The model under review builds one solid part; all positions refer to its coordinate system, in mm. Face numbers are marked on the shaded views. A direction names the side the tool comes from. Coordinates: 2 decimals unless noted, no trailing zeros. Order: outer loops, then holes, each group sorted by start corner. A loop starts at its lowest first (then second) coordinate and runs counter-clockwise, first axis right, second up.
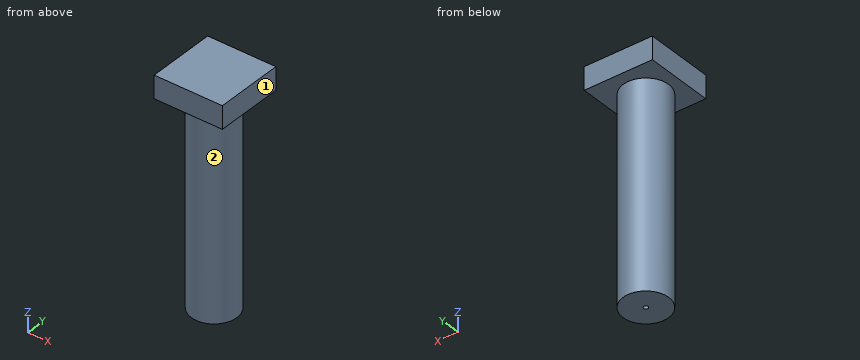
```python
from build123d import *

# Parameters (mm, degrees)
F0_W     = 7.62
F0_H     = 7.62
F1_DEPTH = 2.54
F2_R     = 1.27
F3_DEPTH = 22.86
F4_R     = 0.254
F5_DEPTH = 2.54
F2_R_2   = 2.54
F6_DEPTH = 22.86


# Not quite as in the source:
# - a feature names something its author has since deleted; it is built from what else it names


with BuildPart() as f1:
    # F0 (on Top) → F1 (new body)
    with BuildSketch(Plane.XY):
        with Locations((-38.7955456972, -21.8359371471)):
            Rectangle(F0_W, F0_H)
    extrude(amount=F1_DEPTH)

    # F2 (on face) → F3 (join)
    with BuildSketch(Plane(origin=(0, 0, 0), x_dir=(1, 0, 0), z_dir=(0, 0, -1))):
        with Locations((-38.854431361, 21.8882076442)):
            Circle(F2_R)
    extrude(amount=F3_DEPTH)

    # F4 (on face) → F5 (cut)
    with BuildSketch(Plane(origin=(0, 0, -22.86), x_dir=(1, 0, 0), z_dir=(0, 0, -1))):
        with Locations((-38.854431361, 21.8882076442)):
            Circle(F4_R)
    extrude(amount=-F5_DEPTH, mode=Mode.SUBTRACT)

    # F2 (on face) → F6 (join)
    with BuildSketch(Plane(origin=(0, 0, 0), x_dir=(1, 0, 0), z_dir=(0, 0, -1))):
        with Locations((-38.854431361, 21.8882076442)):
            Circle(F2_R_2)
        with Locations((-38.854431361, 21.8882076442)):
            Circle(F2_R, mode=Mode.SUBTRACT)
    extrude(amount=F6_DEPTH)


solid = f1.part
```
(1) We need section D-D, the plane z = -6.5. Write out the cut boundary in (x, y), and give its area (3 significant figures).
A:
outline: circle Ø5.08 at (-38.85, -21.89)
area: 20.3 mm2
(2) We need section C-C, the plane x = -35.5. Write out the cut boundary in (y, z).
A:
outline: (-25.65, 0) - (-18.03, 0) - (-18.03, 2.54) - (-25.65, 2.54) - close
(3) For pin 1 Ø3 at (x, z) = (-40.5, -8.5) entering from -Y; pin 2 Ø1.5 at (x, y) = (-39, -19) entering from -Z; pin 3 Ø1.5 at (x, z) = (-37.5, -6) entering from +Y; pin 4 Ø4 at (x, z) = (-37, -13.5) entering from +Y, all flat-tipped, find the tip position at first contact; note any pin that passes through.
A:
pin 1: stops at y = -24.42
pin 2: stops at z = -22.86
pin 3: stops at y = -19.42
pin 4: stops at y = -19.35
(4) We need section B-B, the plane y = -19.75. Write out the cut boundary in (x, z).
A:
outline: (-42.61, 0) - (-40.23, 0) - (-40.23, -22.86) - (-37.48, -22.86) - (-37.48, 0) - (-34.99, 0) - (-34.99, 2.54) - (-42.61, 2.54) - close
(5) We need section A-A, the plane x = -37.25. Write out the cut boundary in (y, z), and give its area (3 significant figures).
A:
outline: (-25.65, 0) - (-23.86, 0) - (-23.86, -22.86) - (-19.92, -22.86) - (-19.92, 0) - (-18.03, 0) - (-18.03, 2.54) - (-25.65, 2.54) - close
area: 109 mm2
(6) Wall thickness on probe 1 along Z at (x, y) = (-41.75, -19.75); probe 2 along Y at (x, z) = (-40.25, -6.25); probe 3 along X at (y, z) = (-22.75, -19): over which ranges is each line inside the solid? List them lowest first.
A:
probe 1: z = 0 to 2.54
probe 2: y = -24.01 to -19.77
probe 3: x = -41.24 to -36.47
(7) Machinability: for the marked faces 1 and 2, which of the approach directions +Z, -Z, +X, -X, +Y, -Y give a long, thin tool a straight path to every point of the face, cutting with its end or side? Answer none if there is none.
A:
face 1: +Z, -Z, +X, +Y, -Y
face 2: -Z
